from build123d import *


with BuildPart() as part:
    # Sweep1: sweep along a path in Sketch1
    with BuildLine(Plane(origin=(0, 0, 0), x_dir=(0, 0, -1), z_dir=(1, 0, 0))) as sweep1_path:
        Line((30.24815072, 1.25), (7.806247498, 1.25))
        ThreePointArc((7.806247498, 1.25), (5.641183989, 1.743060906), (3.903123749, 3.125))
        ThreePointArc((3.903123749, 3.125), (-5, 0), (3.903123749, -3.125))
        ThreePointArc((3.903123749, -3.125), (5.641183989, -1.743060906), (7.806247498, -1.25))
        Line((7.806247498, -1.25), (30.24815072, -1.25))
    # Sketch5 → Sweep1 (sweep)
    with BuildSketch(Plane.XY.offset(-30.24815072)):
        with BuildLine():
            Line((-2.292644426, 0.253114081), (2.292644426, 0.253114081))
            ThreePointArc((2.292644426, 0.253114081), (0, 3.75), (-2.292644426, 0.253114081))
        make_face()
    sweep(path=sweep1_path.line)


solid = part.part
Input: part model. Units: mm. Frame: model coordinates. A direction names the side the tool comes from. Round coordinates to 2 decimals unless told otherwise and drop trailing zeros. Loops run counter-clockwise (first coordinate to the right, second up) from the corner with the lowest first, then second, coordinate; pieces in that order, holes last. Notation, with made-up numbers: (62.5, -3) -> (93.5, -3) arc R30 ccw to (93.5, 20) -> close; hole circle Ø6 at (85, 35). An arc over 180 degrees is marked (long way). Answer as a JSON object with one key per item and string values. Group by question number.
1) Section query A-A on x = 0. Output: boundary loops of the cut face in (y, z).
2) Ray query, L1, parallel to Y at x = 0.1, z = -23; L2, parallel to X at y = 2.25, z = -27; L3, parallel to Y at x = -2.1, z = 0. Return the intervals inside material, ascending.
3) Section query C-C on x = 1.8. Output: boundary loops of the cut face in (y, z).
4) Draft query along Z for faces 1 (the flat face through (0, -0.253, -19)), 2 (the cylindrical face through (0, 0.1, 4)), 3 (the flat face through (0, 2, -30.248)), 4 (the cylindrical face through (0.03, -0.86, -5.18)). Return one class per face: +Z half, -Z half, draft (parallel to the pull), parting line (faces both ways), or undercut.
5) Reachability of faces 5 (the cylindrical face through (0.07, -3.75, -19.18)), 6 (the cylindrical face through (0.03, 0.83, -5.24)), 7 (the flat face through (0, 0.253, -19)) from +Z, -Z, +X, -X, +Y, -Y: full face, straight path, thin tool, end or side. Return the list, or none.
6) Pin query (flat end, axial travel): pin 1 (2 mm diameter, centred on y = -4.5, z = -13, fed in from -X); pin 2 (1.5 mm diameter, centred on x = -1, y = 5, fed in from -Z); pin 3 (3 mm diameter, centred on x = 1.5, z = -11.5, fed in from +Y). Return the tip coordinate at first contact, or that it passes through.
7) Section query B-B on z = -25.5. Output: boundary loops of the cut face in (x, y).
Reply:
{
 "1": {"outline": "(-4.69, -5.85) arc R2.5 cw to (-3.75, -7.81) -> (-3.75, -30.25) -> (-0.25, -30.25) -> (-0.25, -7.81) arc R6 ccw to (-2.5, -3.12) arc R4 cw (long way) to (2.5, -3.12) arc R6 ccw to (0.25, -7.81) -> (0.25, -30.25) -> (3.75, -30.25) -> (3.75, -7.81) arc R2.5 cw to (4.69, -5.85) arc R7.5 ccw (long way) to start"},
 "2": {"L1": "y = -3.75 to -0.25, 0.25 to 3.75", "L2": "x = -2.29 to 2.29", "L3": "y = -6.36 to -4, 4 to 6.36"},
 "3": {"outline": "(-4.21, -5.26) arc R3.27 cw to (-2.98, -7.81) -> (-2.98, -30.25) -> (-0.25, -30.25) -> (-0.25, -7.81) arc R6 ccw to (-2.5, -3.12) arc R4 cw (long way) to (2.5, -3.12) arc R6 ccw to (0.25, -7.81) -> (0.25, -30.25) -> (2.98, -30.25) -> (2.98, -7.81) arc R3.27 cw to (4.21, -5.26) arc R6.73 ccw (long way) to start"},
 "4": {"face 1": "draft", "face 2": "undercut", "face 3": "-Z half", "face 4": "undercut"},
 "5": {"face 5": "-Z", "face 6": "+X, -X", "face 7": "-Z, +X, -X"},
 "6": {"pin 1": "stops at x = -1.09", "pin 2": "stops at z = -6.07", "pin 3": "stops at y = 3.75"},
 "7": {"outline": "(-2.29, -0.25) arc R2.5 ccw (long way) to (2.29, -0.25) -> close; (-2.29, 0.25) -> (2.29, 0.25) arc R2.5 ccw (long way) to start"}
}
